Here's how the part is built. I have some questions about the finished solid (model axes, mm). A direction names the side the tool comes from. Coordinates: 2 decimals unless noted, no trailing zeros. Order: outer loops, then holes, each group sorted by start corner. A loop starts at its lowest first (then second) coordinate and runs counter-clockwise, first axis right, second up. Notation, with made-up numbers: (28, 55) - (84, 55) arc R8 cw to (84, 66) - close; hole circle Ø9 at (18.25, 12.25). An arc over 180 degrees is marked (long way). Use CSV: the item, a comma, the result in double quotes. Start each with the question number.
from build123d import *

# Parameters (mm, degrees)
BOSS_EXTRUDE1_DEPTH = 1.8
BOSS_EXTRUDE2_DEPTH = 15
SKETCH3_R           = 4.85
CUT_EXTRUDE1_DEPTH  = 15
SKETCH4_R           = 4.85
CUT_EXTRUDE2_DEPTH  = 15
FILLET1_R           = 3
FILLET2_R           = 4.8
FILLET3_R           = 2
FILLET4_R           = 3.8
BOSS_EXTRUDE3_DEPTH = 1.4
SKETCH6_R           = 2
CUT_EXTRUDE3_DEPTH  = 1.4
BOSS_EXTRUDE4_DEPTH = 1.4
SKETCH8_W           = 41
SKETCH8_H           = 13.6
CUT_EXTRUDE4_DEPTH  = 4.4
FILLET5_R           = 1.8
FILLET6_R           = 3.8


with BuildPart() as part:
    # Sketch1 → Boss-Extrude1 (new body)
    with BuildSketch(Plane.XY):
        Polygon((0, 0), (65, 0), (60, 28), (5, 28), align=None)
    extrude(amount=BOSS_EXTRUDE1_DEPTH)

    # Sketch2 → Boss-Extrude2 (add)
    with BuildSketch(Plane.XY.offset(1.8)):
        Polygon((5, 28), (60, 28), (65, 0), (0, 0), align=None)
        Polygon((6.518195748, 26.4), (58.660404268, 26.4), (63.088975697, 1.6), (2.08962432, 1.6), align=None, mode=Mode.SUBTRACT)
    extrude(amount=BOSS_EXTRUDE2_DEPTH)

    # Sketch3 → Cut-Extrude1 (cut)
    with BuildSketch(Plane(origin=(62.991347342, 11.248454883, 0), x_dir=(0, 0, -1), z_dir=(0.9844275755084821, 0.17579063848365745, 0))):
        with Locations(Location((-8.4, 7.016533805, 0), (0, 0, 90))):
            Circle(SKETCH3_R)
    extrude(amount=-CUT_EXTRUDE1_DEPTH, mode=Mode.SUBTRACT)

    # Sketch4 → Cut-Extrude2 (cut)
    with BuildSketch(Plane(origin=(0, 0, 0), x_dir=(0, 0, 1), z_dir=(-0.9844275755084821, 0.17579063848365759, 0))):
        with Locations(Location((8.4, 18.442925307, 0), (0, 0, 270))):
            Circle(SKETCH4_R)
    extrude(amount=-CUT_EXTRUDE2_DEPTH, mode=Mode.SUBTRACT)

    # Fillet1
    fillet1_edges = [part.edges().sort_by_distance(p)[0] for p in [
        (58.660404268, 26.4, 9.3),
        (6.518195748, 26.4, 9.3),
    ]]
    fillet(fillet1_edges, radius=FILLET1_R)

    # Fillet2
    fillet2_edges = [part.edges().sort_by_distance(p)[0] for p in [
        (5, 28, 8.4),
        (60, 28, 8.4),
    ]]
    fillet(fillet2_edges, radius=FILLET2_R)

    # Fillet3
    fillet3_edges = [part.edges().sort_by_distance(p)[0] for p in [
        (61.095460347, 12.763685958, 1.8),
        (32.589300008, 26.4, 1.8),
        (4.083139669, 12.763685958, 1.8),
        (58.07452367, 25.700229961, 1.8),
        (7.104076347, 25.700229961, 1.8),
    ]]
    fillet(fillet3_edges, radius=FILLET3_R)

    # Fillet4
    # the kernel refuses this fillet: 3.8 mm, written as the material it takes off along each edge
    with BuildSketch(Plane(origin=(55.981212805, 28, 0), x_dir=(0, 0, 1), z_dir=(-1, 0, 0))) as fillet4_piece_1:
        with BuildLine():
            CenterArc((FILLET4_R, -FILLET4_R), FILLET4_R, 90, 90)
            Line((0, -FILLET4_R), (0, 0))
            Line((0, 0), (FILLET4_R, 0))
        make_face()
    extrude(amount=46.962425609, mode=Mode.SUBTRACT)
    with BuildSketch(Plane(origin=(66.670011066, -9.352061967, 0), x_dir=(0, 0, 1), z_dir=(-0.17579063848365728, 0.9844275755084821, 0)), Plane(origin=(4.293534833, 24.043795065, 0), x_dir=(0, 0, 1), z_dir=(-0.17579063848365753, -0.984427575508482, 0))) as fillet4_piece_2:
        with BuildLine():
            CenterArc((FILLET4_R, -FILLET4_R), FILLET4_R, 90, 90)
            Line((0, -FILLET4_R), (0, 0))
            Line((0, 0), (FILLET4_R, 0))
        make_face()
    extrude(amount=33.924138111, mode=Mode.SUBTRACT)
    with BuildSketch(Plane(origin=(9.018787195, 23.2, 0), x_dir=(0, 1, 0), z_dir=(1, 0, 0))) as fillet4_piece_3:
        with BuildLine():
            CenterArc((4.8 - FILLET4_R, FILLET4_R), FILLET4_R, 270, 90)
            Line((4.8 - FILLET4_R, 0), (4.8, 0))
            Line((4.8, 0), (4.8, FILLET4_R))
        make_face()
    revolve(axis=Axis((9.018787195, 23.2, 0), (0, 0, 1)), revolution_arc=79.875328345, mode=Mode.SUBTRACT)
    with BuildSketch(Plane(origin=(55.981212805, 23.2, 0), x_dir=(0, 1, 0), z_dir=(-1, 0, 0))) as fillet4_piece_4:
        with BuildLine():
            CenterArc((4.8 - FILLET4_R, -FILLET4_R), FILLET4_R, 0, 90)
            Line((4.8 - FILLET4_R, 0), (4.8, 0))
            Line((4.8, 0), (4.8, -FILLET4_R))
        make_face()
    revolve(axis=Axis((55.981212805, 23.2, 0), (0, 0, -1)), revolution_arc=79.875328345, mode=Mode.SUBTRACT)

    # Sketch5 → Boss-Extrude3 (add)
    with BuildSketch(Plane.XY.offset(16.8)):
        Polygon((2.08962432, 1.6), (62.853232584, 1.6), (63.866257319, 1.6), (62.171786683, 12.021897532), (3.201344626, 12.021897532), (1.273741814, 1.6), align=None)
    extrude(amount=-BOSS_EXTRUDE3_DEPTH)

    # Sketch6 → Cut-Extrude3 (cut)
    with BuildSketch(Plane.XY.offset(16.8)):
        with Locations((56.933372232, 6.033926522)):
            Circle(SKETCH6_R)
    extrude(amount=-CUT_EXTRUDE3_DEPTH, mode=Mode.SUBTRACT)

    # Sketch7 → Boss-Extrude4 (add)
    with BuildSketch(Plane.XY.offset(16.8)):
        Polygon((6.155527083, 26.711603316), (3.95067745, 17.333364545), (3.95067745, 12.021897532), (61.507859388, 12.021897532), (61.507859388, 17.333364545), (58.93189058, 26.711603316), align=None)
    extrude(amount=-BOSS_EXTRUDE4_DEPTH)

    # Sketch8 → Cut-Extrude4 (cut)
    with BuildSketch(Plane(origin=(0, 0, 0), x_dir=(-1, 0, 0), z_dir=(0, -1, 0))):
        with Locations((-32.5, -8.6)):
            Rectangle(SKETCH8_W, SKETCH8_H)
    extrude(amount=-CUT_EXTRUDE4_DEPTH, mode=Mode.SUBTRACT)

    # Fillet5
    fillet5_edges = [part.edges().sort_by_distance(p)[0] for p in [
        (61.095460347, 12.763685958, 15.4),
        (4.083139669, 12.763685958, 15.4),
        (58.07452367, 25.700229961, 15.4),
        (7.104076347, 25.700229961, 15.4),
        (32.589300008, 26.4, 15.4),
    ]]
    fillet(fillet5_edges, radius=FILLET5_R)

    # Fillet6
    # the kernel refuses this fillet: 3.8 mm, written as the material it takes off along each edge
    with BuildSketch(Plane(origin=(60.706465167, 24.043795065, 16.8), x_dir=(-0.984427575508482, -0.17579063848365725, 0), z_dir=(0.17579063848365728, -0.9844275755084821, 0))) as fillet6_piece_1:
        with BuildLine():
            CenterArc((FILLET6_R, FILLET6_R), FILLET6_R, 180, 90)
            Line((0, FILLET6_R), (0, 0))
            Line((0, 0), (FILLET6_R, 0))
        make_face()
    extrude(amount=33.924138111, mode=Mode.SUBTRACT)
    with BuildSketch(Plane(origin=(9.018787195, 28, 16.8), x_dir=(0, -1, 0), z_dir=(1, 0, 0))) as fillet6_piece_2:
        with BuildLine():
            CenterArc((FILLET6_R, FILLET6_R), FILLET6_R, 180, 90)
            Line((0, FILLET6_R), (0, 0))
            Line((0, 0), (FILLET6_R, 0))
        make_face()
    extrude(amount=46.962425609, mode=Mode.SUBTRACT)
    with BuildSketch(Plane(origin=(-1.670011066, -9.352061967, 16.8), x_dir=(0, 0, -1), z_dir=(0.17579063848365753, 0.984427575508482, 0))) as fillet6_piece_3:
        with BuildLine():
            CenterArc((FILLET6_R, -FILLET6_R), FILLET6_R, 90, 90)
            Line((0, -FILLET6_R), (0, 0))
            Line((0, 0), (FILLET6_R, 0))
        make_face()
    extrude(amount=33.924138111, mode=Mode.SUBTRACT)
    with BuildSketch(Plane(origin=(9.018787195, 23.2, 16.8), x_dir=(0, 1, 0), z_dir=(1, 0, 0))) as fillet6_piece_4:
        with BuildLine():
            CenterArc((4.8 - FILLET6_R, -FILLET6_R), FILLET6_R, 0, 90)
            Line((4.8 - FILLET6_R, 0), (4.8, 0))
            Line((4.8, 0), (4.8, -FILLET6_R))
        make_face()
    revolve(axis=Axis((9.018787195, 23.2, 16.8), (0, 0, 1)), revolution_arc=79.875328345, mode=Mode.SUBTRACT)
    with BuildSketch(Plane(origin=(55.981212805, 23.2, 16.8), x_dir=(0, 1, 0), z_dir=(-1, 0, 0))) as fillet6_piece_5:
        with BuildLine():
            CenterArc((4.8 - FILLET6_R, FILLET6_R), FILLET6_R, 270, 90)
            Line((4.8, FILLET6_R), (4.8, 0))
            Line((4.8, 0), (4.8 - FILLET6_R, 0))
        make_face()
    revolve(axis=Axis((55.981212805, 23.2, 16.8), (0, 0, -1)), revolution_arc=79.875328345, mode=Mode.SUBTRACT)


solid = part.part
Item 1: Suppose I cut it at C-C on z = 10.75. Write out the boundary of the cut face in (x, y), then the cut area to 3 significant figures.
Item 2: For faces 4 (the flat face through (4.158, 23.284, 8.336)), 5 (the cylindrical face through (61.228, 8.777, 2.401)), which set-ups out of +Z, -Z, +X, -X, +Y, -Y let a thin tool reach every point of the face, with its end or its side?
Item 3: Suppose I cut it at A-A on z = 4.5. Write out the boundary of the cut face in (x, y).
Item 4: We'd pull the mould along Z, two halves only. Please class faces 1 (the flat face through (53, 1, 9)), 2 (the cylindrical face through (32.829, 26.916, 1.143)), 3 (the cylindrical face through (3.183, 11.663, 15.657)): released by +Z, released by -Z, zero draft, split by the parting line, or undercut.
Item 5: For pin 1 Ø8 at (x, z) = (43, 8) entering from -Y; pin 2 Ø0.5 at (y, z) = (1, 6) entering from -X; pin 3 Ø3 at (x, z) = (20.5, 13.5) entering from -Y, each with a flat end and sliding along its axis, tell me the tip position at first contact or that it passes through.
Item 6: Suppose I cut it at B-B on x = 34.5. Write out the boundary of the cut face in (y, z).
Item 7: Please list where these lines run through material, in increasing order: line 1 along Z through (x, y) = (43.5, 21.5); line 2 along Y through (x, z) = (54.5, 10.75); line 3 along X through (y, z) = (24.25, 4.25). Write a range as from..to.
Here are the results:
1,outline,"(0, 0) - (12, 0) - (12, 1.6) - (2.09, 1.6) - (4.24, 13.67) - (2.5, 13.98) - close; (3.99, 22.33) - (5.74, 22.02) - (6.08, 23.93) arc R3 cw to (9.03, 26.4) - (56.15, 26.4) arc R3 cw to (59.1, 23.93) - (59.44, 22.05) - (61.01, 22.33) - (60.71, 24.04) arc R4.8 ccw to (55.98, 28) - (9.02, 28) arc R4.8 ccw to (4.29, 24.04) - close; (53, 0) - (65, 0) - (62.5, 13.98) - (60.93, 13.7) - (63.09, 1.6) - (53, 1.6) - close"
1,area,"179 mm^2"
2,face 4,"+Z, -Z, -X, +Y"
2,face 5,"none"
3,outline,"(0, 0) - (12, 0) - (12, 1.6) - (2.09, 1.6) - (4.48, 15.01) - (2.74, 15.32) - close; (3.75, 20.99) - (5.5, 20.68) - (6.08, 23.93) arc R3 cw to (9.03, 26.4) - (56.15, 26.4) arc R3 cw to (59.1, 23.93) - (59.68, 20.71) - (61.25, 20.99) - (60.71, 24.04) arc R4.8 ccw to (55.98, 28) - (9.02, 28) arc R4.8 ccw to (4.29, 24.04) - close; (53, 0) - (65, 0) - (62.26, 15.32) - (60.69, 15.04) - (63.09, 1.6) - (53, 1.6) - close"
4,face 1,"undercut"
4,face 2,"released by -Z"
4,face 3,"released by +Z"
5,pin 1,"y = 26.4"
5,pin 2,"x = 0.13"
5,pin 3,"y = 25.73"
6,outline,"(0, 0) - (24.2, 0) arc R3.8 ccw to (28, 3.8) - (28, 13) arc R3.8 ccw to (24.2, 16.8) - (0, 16.8) - (0, 15.4) - (24.6, 15.4) arc R1.8 cw to (26.4, 13.6) - (26.4, 3.8) arc R2 cw to (24.4, 1.8) - (0, 1.8) - close"
7,line 1,"0..1.8, 15.4..16.8"
7,line 2,"0..1.6, 26.4..28"
7,line 3,"4.34..6.15, 59.03..60.66"
